Read the model definition and answer for the solid it produces. Units are mm, in the model's axes. Coordinates: 2 decimals unless noted, no trailing zeros. Order: outer loops, then holes, each group sorted by start corner. A loop starts at its lowest first (then second) coordinate and runs counter-clockwise, first axis right, second up. Notation, with made-up numbers: (-25.5, 9) -> (30.5, 9) arc R19 ccw to (30.5, 29) -> close; hole circle Ø6 at (40.5, 60). An arc over 180 degrees is marked (long way). Answer as a JSON object with one key per item and string values. Group by question number.
1) Section B-B on z = 0 is taken. Determine the outline of the cut face in (x, y), and give its area (3 significant figures).
2) Section C-C on y = 1.1 is taken. Count the separate pieces of the cut face and the enclosed holes in it, and give its area (3 significant figures).
3) Given pin 1 (2.5 mm diameter, centred on x = 11.22, z = 27.71, fed in from -Y); pin 2 (1.2 mm diameter, centred on y = 2, z = 27.5, fed in from -X); pin 3 (2 mm diameter, centred on y = 2, z = 36.5, fed in from +X); pin 4 (1.2 mm diameter, centred on x = -7.5, y = 2.5, fed in from -Z), each flat-ended and moving along its own axis, determine where each tip first touches the part or whether it passes through.
4) Section D-D on z = -16 is taken. Determine the outline of the cut face in (x, y).
5) Consider L1, parallel to Z at x = -6, y = 1.1; L2, parallel to Z at x = -0.5, y = 3.45; L3, parallel to Z at x = 16.5, y = 1.65. Determine where each line is inside the solid, lowest interval first.
6) Section A-A on z = 18 is taken. Determine the outline of the cut face in (x, y).
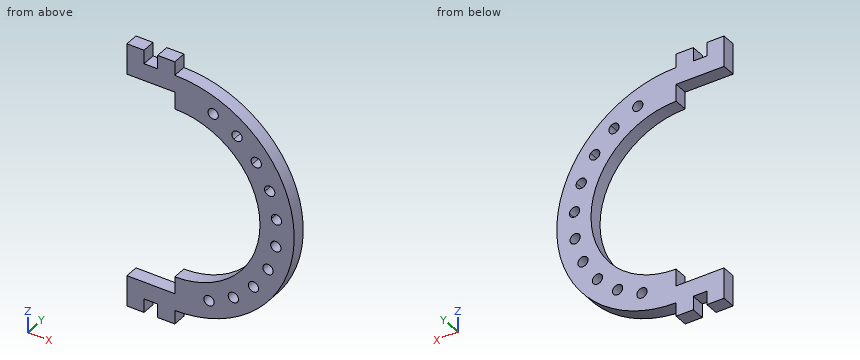
from build123d import *

# Parameters (mm, degrees)
BOSS_EXTRUDE1_DEPTH = 4
SKETCH2_W           = 5
SKETCH2_H           = 4
BOSS_EXTRUDE2_DEPTH = 4
SKETCH3_R           = 1.5
CUT_EXTRUDE1_DEPTH  = 53.413929446
CIRPATTERN2_COUNT   = 9
CIRPATTERN2_ANGLE   = 123.04


with BuildPart() as part:
    # Sketch1 → Boss-Extrude1 (new body)
    with BuildSketch(Plane(origin=(0, 0, 0), x_dir=(1, 0, 0), z_dir=(0, 1, 0))):
        with BuildLine():
            ThreePointArc((0, -34.9), (34.9, 0), (0, 34.9))
            Line((0, 34.9), (0, 24.9))
            ThreePointArc((0, 24.9), (24.9, 0), (0, -24.9))
            Line((0, -24.9), (0, -34.9))
        make_face()
    extrude(amount=BOSS_EXTRUDE1_DEPTH)

    # Sketch2 → Boss-Extrude2 (add, through all)
    with BuildSketch(Plane(origin=(0, 4, 0), x_dir=(1, 0, 0), z_dir=(0, 1, 0))):
        with Locations((-11.5, 36.9)):
            Rectangle(SKETCH2_W, SKETCH2_H)
        Polygon((-14, 29.9), (0, 29.9), (0, 34.9), (-5, 34.9), (-9, 34.9), (-14, 34.9), align=None)
        with Locations((-2.5, 36.9)):
            Rectangle(SKETCH2_W, SKETCH2_H)
        Polygon((-9, -34.9), (-5, -34.9), (0, -34.9), (0, -29.9), (-14, -29.9), (-14, -34.9), align=None)
        with Locations((-11.5, -36.9)):
            Rectangle(SKETCH2_W, SKETCH2_H)
        with Locations((-2.5, -36.9)):
            Rectangle(SKETCH2_W, SKETCH2_H)
    extrude(amount=-BOSS_EXTRUDE2_DEPTH)

    # Sketch3 → Cut-Extrude1 (cut, through all)
    with BuildSketch(Plane(origin=(0, 4, 0), x_dir=(1, 0, 0), z_dir=(0, 1, 0))):
        with Locations(Location((10, 28.17818305, 0), (0, 0, 270))):
            Circle(SKETCH3_R)
        with Locations(Location((17.113605639, 24.518044417, 0), (0, 0, 270))):
            Circle(SKETCH3_R)
    cut_extrude1 = extrude(amount=-CUT_EXTRUDE1_DEPTH, mode=Mode.SUBTRACT)

    # CirPattern2: Cut-Extrude1 ×9 about axis
    cirpattern2_axis = Axis((0, 0, 0), (0, -1, 0))
    for i in range(1, CIRPATTERN2_COUNT):
        add(cut_extrude1.rotate(cirpattern2_axis, i * CIRPATTERN2_ANGLE / (CIRPATTERN2_COUNT - 1)), mode=Mode.SUBTRACT)


solid = part.part
Worked answers:
{
 "1": {"outline": "(24.9, 0) -> (34.9, 0) -> (34.9, 4) -> (24.9, 4) -> close", "area": "40.0 mm²"},
 "2": {"separate pieces": "1", "enclosed holes": "10", "area": "1,090 mm²"},
 "3": {"pin 1": "passes through", "pin 2": "stops at x = 0", "pin 3": "stops at x = 0", "pin 4": "stops at z = -34.9"},
 "4": {"outline": "(19.08, 0) -> (31.02, 0) -> (31.02, 4) -> (19.08, 4) -> close"},
 "5": {"L1": "z = -34.9 to -29.9, 29.9 to 34.9", "L2": "z = -38.9 to -29.9, 29.9 to 38.9", "L3": "z = -30.75 to -25.89, -23.15 to -18.65, 18.65 to 30.75"},
 "6": {"outline": "(17.2, 0) -> (22.32, 0) -> (22.32, 4) -> (17.2, 4) -> close; (25.32, 0) -> (29.9, 0) -> (29.9, 4) -> (25.32, 4) -> close"}
}
